```python
from build123d import *

# Parameters (mm, degrees)
F0_W     = 920
F0_H     = 120
F1_DEPTH = 21
F2_SIZE  = 20
F3_SIZE  = 119.99999


# Not quite as in the source:
# - a fillet or chamfer is up to 0.001 mm smaller than in the source, because OpenCascade refuses the exact size


with BuildPart() as f1:
    # F0 (on Top) → F1 (new body)
    with BuildSketch(Plane.XY):
        Rectangle(F0_W, F0_H)
    extrude(amount=F1_DEPTH)

    # F2
    f2_edges = [f1.edges().sort_by_distance(p)[0] for p in [
        (-460, 60, 10.5),
        (-460, -60, 10.5),
    ]]
    chamfer(f2_edges, length=F2_SIZE)

    # F3 (size 120 in the source; OpenCascade refuses exactly that, so slightly less here)
    f3_edges = [f1.edges().sort_by_distance(p)[0] for p in [
        (460, -60, 10.5),
    ]]
    chamfer(f3_edges, length=F3_SIZE)


solid = f1.part
```
For this review, take the finished solid that the model builds, in its own axes (mm). Give positions to 0.01 mm unless a question says otherwise; leave off trailing zeros. Order: outer loops, then holes, each group sorted by start corner. A loop starts at its lowest first (then second) coordinate and runs counter-clockwise, first axis right, second up.
1) Insertion check: pin 1 (1.5 mm diameter, centred on y = 44.5, z = 2.5, fed in from +X); pin 2 (2 mm diameter, centred on y = -39.5, z = 9, fed in from +X); pin 3 (5 mm diameter, centred on y = 44, z = 16, fed in from -X). Each pin has a flat end and moves straight along its axis. Give the tip position at first contact, or say it passes through.
2) Wall thickness on line 1 (X direction, y = -16, z = 13.5); line 2 (X direction, y = -1.5, z = 14): over which ranges is each line inside the solid? List them lowest first.
3) Take a section at C-C (y = -19). Give the boundary of the cut face in (x, z), then the cut area to 3 significant figures.
4) Take a section at B-B (y = 26.5). Give the boundary of the cut face in (x, z).
Derived:
1. pin 1: stops at x = 445.25
1. pin 2: stops at x = 361.5
1. pin 3: stops at x = -458.5
2. line 1: x = -460 to 384
2. line 2: x = -460 to 398.5
3. outline: (-460, 0) - (381, 0) - (381, 21) - (-460, 21) - close
3. area: 17,700 mm2
4. outline: (-460, 0) - (426.5, 0) - (426.5, 21) - (-460, 21) - close
